```python
from build123d import *

# Parameters (mm, degrees)
F0_R     = 4.8895
F1_DEPTH = 6.35


with BuildPart() as f1:
    # F0 (on Front) → F1 (new body)
    with BuildSketch(Plane.XZ):
        with BuildLine():
            ThreePointArc((-76.2, -76.2), (-68.760512, -94.160512), (-50.8, -101.6))
            Line((-50.8, -101.6), (50.8, -101.6))
            ThreePointArc((50.8, -101.6), (68.760512, -94.160512), (76.2, -76.2))
            Line((76.2, -76.2), (76.2, 76.2))
            ThreePointArc((76.2, 76.2), (68.760512, 94.160512), (50.8, 101.6))
            Line((50.8, 101.6), (-50.8, 101.6))
            ThreePointArc((-50.8, 101.6), (-68.760512, 94.160512), (-76.2, 76.2))
            Line((-76.2, 76.2), (-76.2, -76.2))
        make_face()
        with Locations((-50.8, -76.2)):
            Circle(F0_R, mode=Mode.SUBTRACT)
        with BuildLine():
            Line((3.3655, -69.85), (-3.3655, -69.85))
            ThreePointArc((-3.3655, -69.85), (-3.590006, -69.757006), (-3.683, -69.5325))
            Line((-3.683, -69.5325), (-3.683, 69.5325))
            ThreePointArc((-3.683, 69.5325), (-3.590006, 69.757006), (-3.3655, 69.85))
            Line((-3.3655, 69.85), (3.3655, 69.85))
            ThreePointArc((3.3655, 69.85), (3.590006, 69.757006), (3.683, 69.5325))
            Line((3.683, 69.5325), (3.683, -69.5325))
            ThreePointArc((3.683, -69.5325), (3.590006, -69.757006), (3.3655, -69.85))
        make_face(mode=Mode.SUBTRACT)
        with Locations((50.8, -76.2)):
            Circle(F0_R, mode=Mode.SUBTRACT)
        with Locations((-50.8, 76.2)):
            Circle(F0_R, mode=Mode.SUBTRACT)
        with Locations((50.8, 76.2)):
            Circle(F0_R, mode=Mode.SUBTRACT)
    extrude(amount=F1_DEPTH)


solid = f1.part
```
Input: part model. Units: mm. Frame: model coordinates. A direction names the side the tool comes from. Coordinates: 2 decimals unless noted, no trailing zeros. Write each loop counter-clockwise with the first axis right and the second up, starting at its lowest first coordinate (ties: lowest second). Pieces come first, ordered by that corner, then holes. Notation, with made-up numbers: (7, 37) - (66, 37) arc R21 ccw to (66, 70) - close; hole circle Ø1 at (-24.75, -35). An arc over 180 degrees is marked (long way). Put each result on its own line as item: value. Start each with the question number.
1) Cut plane B-B (y = -2.25). State how many separate pieces and enclosed holes the cut face has, plus the area to 3 significant figures.
2) Mould query, pull axis X, two halves, no side actions, for faces 1 (the face through (3.683, -3, 1)), 2 (the face through (76.2, -3, -1)), 3 (the face through (-68.56, -3.13, 94.36)). Classes: pulls with the +X half, pulls with the -X half, needs draft (parallel to the pull), parting line crosses it, or undercut.
3) Reachability of faces 4 (the face through (0, -3, -69.85)), 5 (the face through (68.96, -3.13, 93.96)) from +Z, -Z, +X, -X, +Y, -Y: full face, straight path, thin tool, end or side. Return the list, or none.
4) Cut plane C-C (x = -65). Return the cut outline in (y, z), plus the area to 3 significant figures.
5) Cut plane A-A (z = 62.5). Return the cut outline in (x, y).
6) Contact query for flat-ended pins moving along their axis: pin 1 (9 mm diameter, centred on x = -50.8, z = 76.2, fed in from +Y); pin 2 (2 mm diameter, centred on x = 54, y = -1, fed in from -Z); pin 3 (1.5 mm diameter, centred on x = -58.5, y = -1, fed in from -Z). Output: stop coordinate, or through.
7) Ray query, L1, parallel to Z at x = 50.8, y = -3.5; L2, parallel to X at y = -4, z = 52; L3, parallel to Z at x = -3.5, y = -3. Return the intervals inside material, ascending.
Resolved:
1. separate pieces: 1
1. enclosed holes: 5
1. area: 29,100 mm2
2. face 1: undercut
2. face 2: pulls with the +X half
2. face 3: pulls with the -X half
3. face 4: +Y, -Y
3. face 5: +Z, +X, +Y, -Y
4. outline: (-6.35, -97.26) - (0, -97.26) - (0, 97.26) - (-6.35, 97.26) - close
4. area: 1,240 mm2
5. outline: (-76.2, -6.35) - (-3.68, -6.35) - (-3.68, 0) - (-76.2, 0) - close; (3.68, -6.35) - (76.2, -6.35) - (76.2, 0) - (3.68, 0) - close
6. pin 1: passes through
6. pin 2: stops at z = -101.5
6. pin 3: stops at z = -100.63
7. L1: z = -101.6 to -81.09, -71.31 to 71.31, 81.09 to 101.6
7. L2: x = -76.2 to -3.68, 3.68 to 76.2
7. L3: z = -101.6 to -69.82, 69.82 to 101.6
